from build123d import *

# Parameters (mm, degrees)
EXTRUDE_1_DEPTH     = 9
CUT_EXTRUDE_2_DEPTH = 68.284842275
SKETCH_6_W          = 5
SKETCH_6_H          = 25
CUT_EXTRUDE_3_DEPTH = 67.927199254
FILLET_1_R          = 3
SKETCH_7_W          = 6.5
SKETCH_7_H          = 4
EXTRUDE_2_DEPTH     = 9
FILLET_2_R          = 2


with BuildPart() as part:
    # Эскиз1 → Бобышка-Вытянуть1 (new body)
    with BuildSketch(Plane.XY):
        Polygon((0, 0), (9.5, 0), (9.5, 3), (3, 3), (3, 66), (0, 66), align=None)
    extrude(amount=EXTRUDE_1_DEPTH)

    # Эскиз4 → Вырез-Вытянуть2 (cut, through all)
    with BuildSketch(Plane.ZY):
        with BuildLine():
            Line((6.25, 55.52), (6.25, 49.52))
            ThreePointArc((6.25, 49.52), (4.5, 47.77), (2.75, 49.52))
            Line((2.75, 49.52), (2.75, 55.52))
            ThreePointArc((2.75, 55.52), (4.5, 57.27), (6.25, 55.52))
        make_face()
    extrude(amount=-CUT_EXTRUDE_2_DEPTH, mode=Mode.SUBTRACT)

    # Эскиз6 → Вырез-Вытянуть3 (cut, through all)
    with BuildSketch(Plane(origin=(3, 0, 0), x_dir=(0, 0, -1), z_dir=(1, 0, 0))):
        with Locations((-4.5, 18.5)):
            Rectangle(SKETCH_6_W, SKETCH_6_H)
    extrude(amount=-CUT_EXTRUDE_3_DEPTH, mode=Mode.SUBTRACT)

    # Скругление1
    fillet_1_edges = [part.edges().sort_by_distance(p)[0] for p in [
        (3, 3, 4.5),
    ]]
    fillet(fillet_1_edges, radius=FILLET_1_R - 0.0001)  # a hair under: the kernel refuses the full size

    # Эскиз7 → Бобышка-Вытянуть2 (add)
    with BuildSketch(Plane.XY.offset(9)):
        with Locations((6.25, 37)):
            Rectangle(SKETCH_7_W, SKETCH_7_H)
    extrude(amount=-EXTRUDE_2_DEPTH)

    # Скругление2
    fillet_2_edges = [part.edges().sort_by_distance(p)[0] for p in [
        (3, 39, 4.5),
        (3, 35, 4.5),
    ]]
    fillet(fillet_2_edges, radius=FILLET_2_R)


solid = part.part
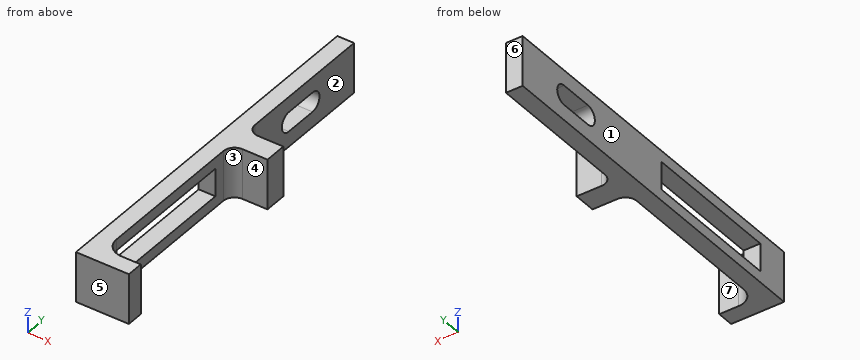
Build history of the part. All positions in model axes, mm. Face numbers are marked on the shaded views. A direction names the side the tool comes from. Give positions to 0.01 mm unless a question says otherwise; leave off trailing zeros. Write each loop counter-clockwise with the first axis right and the second up, starting at its lowest first coordinate (ties: lowest second). Pieces come first, ordered by that corner, then holes. Notation, with made-up numbers: (88, 10) - (118, 10) arc R17 ccw to (118, 36) - close; hole circle Ø11 at (61, 49). An arc over 180 degrees is marked (long way). Use one line per item in the form item = value. Start each with the question number.
1. Probe line 1 (Y direction, x = 7.75, z = 8); line 2 (Y direction, x = 2.25, z = 5.25); line 3 (Z direction, x = 1.25, y = 23.5). List the from-to ranges inside material, lowest first. Write a range as [from, to].
2. 3-axis set-ups, long thin cutter, end or side, ignore diameter. For the marked faces 1, 2 and 3: which of +Z, -Z, +X, -X, +Y, -Y reach the whole face in a straight line?
3. Two-plate mould, pull along Y, no slides. Class the marked faces 4, 5, 6 and 7: released by +Y, released by -Y, zero draft, split by the parting line, or undercut.
4. Band-saw the part on B-B on x = 8.75. Write the cut outline in (y, z), plus the area to 3 significant figures.
5. Band-saw the part on A-A on y = 7. Write the cut outline in (x, z), plus the area to 3 significant figures.
6. Drop flat-ended pins along their axis: pin 1 Ø1.3 at (x, z) = (7, 4) entering from +Y; pin 2 Ø4 at (x, y) = (6, 28) entering from -Z (3 decimals); pin 3 Ø4 at (y, z) = (21.5, 1.5) entering from +X. Give the stop position or say it passes through.
7. Band-saw the part on C-C on z = 4.5. Count the separate pieces of the cut face and the enclosed holes in it, plus the area to 3 significant figures.
8. Band-saw the part on D-D on x = 2. Write the cut outline in (y, z), plus the area to 3 significant figures.
Conclusion:
q1.line_1 = [0, 3], [35, 39]
q1.line_2 = [0, 6], [31, 47.94], [57.1, 66]
q1.line_3 = [0, 2], [7, 9]
q2.face_1 = +Z, -Z, -X, +Y, -Y
q2.face_2 = +Z, -Z, +X, +Y
q2.face_3 = +Z, -Z, +X
q3.face_4 = undercut
q3.face_5 = released by -Y
q3.face_6 = released by +Y
q3.face_7 = undercut
q4.outline = (0, 0) - (3, 0) - (3, 9) - (0, 9) - close; (35, 0) - (39, 0) - (39, 9) - (35, 9) - close
q4.area = 63.0 mm²
q5.outline = (0, 0) - (3, 0) - (3, 2) - (0, 2) - close; (0, 7) - (3, 7) - (3, 9) - (0, 9) - close
q5.area = 12.0 mm²
q6.pin_1 = 39
q6.pin_2 = through
q6.pin_3 = 3
q7.separate_pieces = 3
q7.enclosed_holes = 0
q7.area = 144 mm²
q8.outline = (0, 0) - (66, 0) - (66, 9) - (0, 9) - close; hole (6, 2) - (31, 2) - (31, 7) - (6, 7) - close; hole (49.52, 2.75) - (55.52, 2.75) arc R1.75 ccw to (55.52, 6.25) - (49.52, 6.25) arc R1.75 ccw to start
q8.area = 438 mm²
